Work out the finished part from the listing and answer in its coordinate system (mm). Coordinates: 2 decimals unless noted, no trailing zeros. Order: outer loops, then holes, each group sorted by start corner. A loop starts at its lowest first (then second) coordinate and runs counter-clockwise, first axis right, second up.
```python
from build123d import *

# Parameters (mm, degrees)
SKETCH1_W                      = 861.06
SKETCH1_H                      = 63.5
BASE_FLANGE1_DEPTH             = 1.89738
EDGE_FLANGE1_STRIP_W           = 12.66952
EDGE_FLANGE1_STRIP_H           = 1.89738
EDGE_FLANGE1_STRIP_CUT_DEPTH   = 861.06
EDGE_FLANGE1_STRIP_2_W         = 12.66952
EDGE_FLANGE1_STRIP_2_H         = 1.89738
EDGE_FLANGE1_STRIP_CUT_2_DEPTH = 861.06
EDGE_FLANGE1_DEPTH             = 861.06
EDGE_FLANGE1_BEND_DEPTH        = 861.06
SKETCH12_W                     = 1.89738
SKETCH12_H                     = 54.62524
BOSS_EXTRUDE1_DEPTH            = 24.765
EDGE_FLANGE2_STRIP_W           = 12.66952
EDGE_FLANGE2_STRIP_H           = 1.89738
EDGE_FLANGE2_STRIP_CUT_DEPTH   = 54.62524
EDGE_FLANGE2_STRIP_2_W         = 12.66952
EDGE_FLANGE2_STRIP_2_H         = 1.89738
EDGE_FLANGE2_STRIP_CUT_2_DEPTH = 54.62524
EDGE_FLANGE2_DEPTH             = 54.62524
EDGE_FLANGE2_BEND_DEPTH        = 54.62524
SKETCH16_W                     = 9.525
SKETCH16_H                     = 50.8
CUT_EXTRUDE1_DEPTH             = 4.7752
LPATTERN1_COUNT                = 3
LPATTERN1_PITCH                = 381
SKETCH17_R                     = 3.3655
CUT_EXTRUDE2_DEPTH             = 2.54
CUT_EXTRUDE3_DEPTH             = 2.54
LPATTERN2_COUNT                = 2
LPATTERN2_PITCH                = 482.6
SKETCH25_R                     = 2.4638
CUT_EXTRUDE4_DEPTH             = 914.154728455
CHAMFER1_SIZE                  = 2.54


# Sheet-metal steps are written as plain solids
with BuildPart() as part:
    # Sketch1 → Base-Flange1 (new body)
    with BuildSketch(Plane(origin=(0, 0, 0), x_dir=(0, 0, -1), z_dir=(1, 0, 0))):
        with Locations((430.53, 31.75)):
            Rectangle(SKETCH1_W, SKETCH1_H)
    extrude(amount=-BASE_FLANGE1_DEPTH)

    # Edge-Flange1 strip (across the edge) → Edge-Flange1 strip cut (cut)
    with BuildSketch(Plane(origin=(-1.89738, 63.5, 0), x_dir=(0, -1, 0), z_dir=(0, 0, -1))):
        with Locations((-1.89738, -0.94869)):
            Rectangle(EDGE_FLANGE1_STRIP_W, EDGE_FLANGE1_STRIP_H)
    extrude(amount=EDGE_FLANGE1_STRIP_CUT_DEPTH, mode=Mode.SUBTRACT)

    # Edge-Flange1 strip 2 (across the edge) → Edge-Flange1 strip cut 2 (cut)
    with BuildSketch(Plane(origin=(-1.89738, 0, -861.06), x_dir=(0, 1, 0), z_dir=(0, 0, 1))):
        with Locations((-1.89738, -0.94869)):
            Rectangle(EDGE_FLANGE1_STRIP_2_W, EDGE_FLANGE1_STRIP_2_H)
    extrude(amount=EDGE_FLANGE1_STRIP_CUT_2_DEPTH, mode=Mode.SUBTRACT)

    # Edge-Flange1 section (across the edge) → Edge-Flange1 (add)
    with BuildSketch(Plane(origin=(-1.89738, 63.5, 0), x_dir=(0, -1, 0), z_dir=(0, 0, -1))):
        with BuildLine():
            Line((0, 2.54), (0, 23.50262))
            Line((0, 23.50262), (1.89738, 23.50262))
            Line((1.89738, 23.50262), (1.89738, 2.54))
            ThreePointArc((1.89738, 2.54), (2.641328776, 0.743948776), (4.43738, 0))
            Line((4.43738, 0), (4.43738, -1.89738))
            ThreePointArc((4.43738, -1.89738), (1.299678511, -0.597701489), (0, 2.54))
        make_face()
    extrude(amount=EDGE_FLANGE1_DEPTH)

    # Edge-Flange1 section 2 (across the edge) → Edge-Flange1 bend (add)
    with BuildSketch(Plane(origin=(-1.89738, 0, -861.06), x_dir=(0, 1, 0), z_dir=(0, 0, 1))):
        with BuildLine():
            Line((0, 2.54), (0, 23.50262))
            Line((0, 23.50262), (1.89738, 23.50262))
            Line((1.89738, 23.50262), (1.89738, 2.54))
            ThreePointArc((1.89738, 2.54), (2.641328776, 0.743948776), (4.43738, 0))
            Line((4.43738, 0), (4.43738, -1.89738))
            ThreePointArc((4.43738, -1.89738), (1.299678511, -0.597701489), (0, 2.54))
        make_face()
    extrude(amount=EDGE_FLANGE1_BEND_DEPTH)

    # Sketch12 → Boss-Extrude1 (add)
    with BuildSketch(Plane.XY):
        with Locations((-0.94869, 31.75)):
            Rectangle(SKETCH12_W, SKETCH12_H)
    boss_extrude1 = extrude(amount=BOSS_EXTRUDE1_DEPTH)

    # Mirror1: Boss-Extrude1 across plane
    add(boss_extrude1.mirror(Plane.XY.offset(-430.53)))

    # Edge-Flange2 strip (across the edge) → Edge-Flange2 strip cut (cut)
    with BuildSketch(Plane(origin=(-1.89738, 4.43738, 24.765), x_dir=(0, 0, -1), z_dir=(0, 1, 0))):
        with Locations((-1.89738, -0.94869)):
            Rectangle(EDGE_FLANGE2_STRIP_W, EDGE_FLANGE2_STRIP_H)
    extrude(amount=EDGE_FLANGE2_STRIP_CUT_DEPTH, mode=Mode.SUBTRACT)

    # Edge-Flange2 strip 2 (across the edge) → Edge-Flange2 strip cut 2 (cut)
    with BuildSketch(Plane(origin=(-1.89738, 59.06262, -885.825), x_dir=(0, 0, 1), z_dir=(0, -1, 0))):
        with Locations((-1.89738, -0.94869)):
            Rectangle(EDGE_FLANGE2_STRIP_2_W, EDGE_FLANGE2_STRIP_2_H)
    extrude(amount=EDGE_FLANGE2_STRIP_CUT_2_DEPTH, mode=Mode.SUBTRACT)

    # Edge-Flange2 section (across the edge) → Edge-Flange2 (add)
    with BuildSketch(Plane(origin=(-1.89738, 4.43738, 24.765), x_dir=(0, 0, -1), z_dir=(0, 1, 0))):
        with BuildLine():
            Line((0, 2.54), (0, 23.50262))
            Line((0, 23.50262), (1.89738, 23.50262))
            Line((1.89738, 23.50262), (1.89738, 2.54))
            ThreePointArc((1.89738, 2.54), (2.641328776, 0.743948776), (4.43738, 0))
            Line((4.43738, 0), (4.43738, -1.89738))
            ThreePointArc((4.43738, -1.89738), (1.299678511, -0.597701489), (0, 2.54))
        make_face()
    extrude(amount=EDGE_FLANGE2_DEPTH)

    # Edge-Flange2 section 2 (across the edge) → Edge-Flange2 bend (add)
    with BuildSketch(Plane(origin=(-1.89738, 59.06262, -885.825), x_dir=(0, 0, 1), z_dir=(0, -1, 0))):
        with BuildLine():
            Line((0, 2.54), (0, 23.50262))
            Line((0, 23.50262), (1.89738, 23.50262))
            Line((1.89738, 23.50262), (1.89738, 2.54))
            ThreePointArc((1.89738, 2.54), (2.641328776, 0.743948776), (4.43738, 0))
            Line((4.43738, 0), (4.43738, -1.89738))
            ThreePointArc((4.43738, -1.89738), (1.299678511, -0.597701489), (0, 2.54))
        make_face()
    extrude(amount=EDGE_FLANGE2_BEND_DEPTH)

    # Sketch16 → Cut-Extrude1 (cut)
    with BuildSketch(Plane(origin=(0, 63.5, 0), x_dir=(1, 0, 0), z_dir=(0, 1, 0))):
        with Locations((-4.7625, 49.53)):
            Rectangle(SKETCH16_W, SKETCH16_H)
    cut_extrude1 = extrude(amount=-CUT_EXTRUDE1_DEPTH, mode=Mode.SUBTRACT)

    # LPattern1: Cut-Extrude1 ×3
    with Locations(*[(0, 0, -i * LPATTERN1_PITCH) for i in range(1, LPATTERN1_COUNT)]):
        add(cut_extrude1, mode=Mode.SUBTRACT)

    # Sketch17 → Cut-Extrude2 (cut)
    with BuildSketch(Plane(origin=(0, 63.5, 0), x_dir=(1, 0, 0), z_dir=(0, 1, 0))):
        with Locations(Location((-12.7, 481.33, 0), (0, 0, 180))):
            Circle(SKETCH17_R)
        with Locations(Location((-12.7, 379.73, 0), (0, 0, 180))):
            Circle(SKETCH17_R)
    extrude(amount=-CUT_EXTRUDE2_DEPTH, mode=Mode.SUBTRACT)

    # Sketch18 → Cut-Extrude3 (cut)
    with BuildSketch(Plane(origin=(0, 0, 0), x_dir=(0, 0, -1), z_dir=(1, 0, 0))):
        with BuildLine():
            Line((125.73, 47.625), (252.73, 47.625))
            ThreePointArc((252.73, 47.625), (268.605, 31.75), (252.73, 15.875))
            Line((252.73, 15.875), (125.73, 15.875))
            ThreePointArc((125.73, 15.875), (109.855, 31.75), (125.73, 47.625))
        make_face()
    cut_extrude3 = extrude(amount=-CUT_EXTRUDE3_DEPTH, mode=Mode.SUBTRACT)

    # LPattern2: Cut-Extrude3 ×2
    with Locations(*[(0, 0, -i * LPATTERN2_PITCH) for i in range(1, LPATTERN2_COUNT)]):
        add(cut_extrude3, mode=Mode.SUBTRACT)

    # Sketch25 → Cut-Extrude4 (cut, through all)
    with BuildSketch(Plane.XY.offset(24.765)):
        with Locations((-12.7, 50.8)):
            Circle(SKETCH25_R)
        with Locations((-12.7, 12.7)):
            Circle(SKETCH25_R)
    extrude(amount=-CUT_EXTRUDE4_DEPTH, mode=Mode.SUBTRACT)

    # Chamfer1
    chamfer1_edges = [part.edges().sort_by_distance(p)[0] for p in [
        (-25.4, 4.43738, 23.81631),
        (-25.4, 59.06262, 23.81631),
        (-25.4, 59.06262, -884.87631),
        (-25.4, 4.43738, -884.87631),
        (-25.4, 62.55131, 0),
        (-25.4, 62.55131, -861.06),
        (-25.4, 0.94869, -861.06),
        (-25.4, 0.94869, 0),
    ]]
    chamfer(chamfer1_edges, length=CHAMFER1_SIZE)


solid = part.part
```
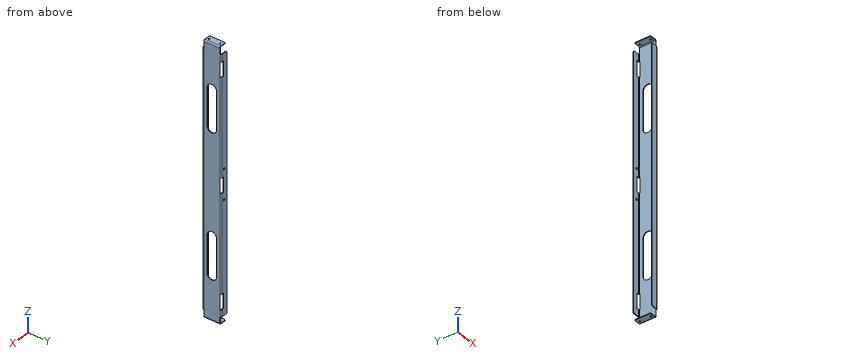
1. Flat-ended cylindrical pins translate along their axes: pin 1 (11.5 mm diameter, centred on x = -11.5, z = -878.5, fed in from -Y); pin 2 (1.5 mm diameter, centred on x = -1, z = -211.5, fed in from +Y); pin 3 (0.6 mm diameter, centred on y = 62.5, z = -423, fed in from +X) (3 decimals). Find the tip coordinate at first contact, or state that the pin passes through.
2. The part is cut by section B-B (y = 31.75). Determine the outline of the cut face in (x, z) (3 decimals).
3. The part is cut by section C-C (z = -807.5). Determine the outline of the cut face in (x, y) (3 decimals).
4. The part is cut by section A-A (z = -143). Determine the outline of the cut face in (x, y) (3 decimals), plus the area to 3 significant figures.
5. Consider probe 1 along Y at (x, z) = (-12.7, -884.7); probe 2 along Z at (x, y) = (-12.7, 62.4); probe 3 along Z at (x, y) = (-7.75, 6) (3 decimals). Determine where each line is inside the solid, lowest interval first.
Worked out:
1. pin 1: stops at y = 4.44
1. pin 2: stops at y = 62.59
1. pin 3: stops at x = -9.525
2. outline: (-25.4, -885.825) - (-4.437, -885.825) arc R4.437 ccw to (0, -881.388) - (0, -751.205) - (-1.897, -751.205) - (-1.897, -881.388) arc R2.54 cw to (-4.437, -883.928) - (-25.4, -883.928) - close; (-25.4, 22.868) - (-4.437, 22.868) arc R2.54 cw to (-1.897, 20.328) - (-1.897, -109.855) - (0, -109.855) - (0, 20.328) arc R4.437 ccw to (-4.437, 24.765) - (-25.4, 24.765) - close; (-1.897, -592.455) - (0, -592.455) - (0, -268.605) - (-1.897, -268.605) - close
3. outline: (-25.4, 0) - (-4.437, 0) arc R4.437 ccw to (0, 4.437) - (0, 58.725) - (-1.897, 58.725) - (-1.897, 4.437) arc R2.54 cw to (-4.437, 1.897) - (-25.4, 1.897) - close; (-25.4, 61.603) - (-9.525, 61.603) - (-9.525, 63.5) - (-25.4, 63.5) - close
4. outline: (-25.4, 0) - (-4.437, 0) arc R4.437 ccw to (0, 4.437) - (0, 15.875) - (-1.897, 15.875) - (-1.897, 4.437) arc R2.54 cw to (-4.437, 1.897) - (-25.4, 1.897) - close; (-25.4, 61.603) - (-4.437, 61.603) arc R2.54 cw to (-1.897, 59.063) - (-1.897, 47.625) - (0, 47.625) - (0, 59.063) arc R4.437 ccw to (-4.437, 63.5) - (-25.4, 63.5) - close
4. area: 144 mm2
5. probe 1: y = 4.44 to 10.24, 15.16 to 48.34, 53.26 to 59.06
5. probe 2: z = -861.06 to -484.7, -477.96 to -383.1, -376.36 to 0
5. probe 3: z = -885.825 to -883.928, 22.868 to 24.765
